Input: part model. Units: mm. Frame: model coordinates. Coordinates: 2 decimals unless noted, no trailing zeros. Write each loop counter-clockwise with the first axis right and the second up, starting at its lowest first coordinate (ties: lowest second). Pieces come first, ordered by that corner, then holes. Notation, with made-up numbers: (5, 29) - (54, 29) arc R17 cw to (54, 48) - close; hole circle Ø6 at (82, 3). An arc over 180 degrees is marked (long way). Put each result on its own line as item: value. Start each with the question number.
1. Cut plane B-B, the plane z = 6. Return loops of the section in (x, y).
2. Cut plane C-C, the plane x = 6. Return loops of the section in (y, z), and give its area (3 significant figures).
3. Cut plane A-A, the plane y = -13.5. Return loops of the section in (x, z).
4. Pin query (flat end, axial travel): pin 1 (1.5 mm diameter, centred on y = -30.5, z = 4.5, fed in from -X). Return the tip coordinate at first contact, or that it passes through.
5. Line query: line 1 (Z direction, x = -0.25, y = -7.5); line 2 (Z direction, x = 7.5, y = -33.5); line 3 (X direction, y = -27, z = 2.5). Output: solid intervals per line, ascending.
from build123d import *

# Parameters (mm, degrees)
F1_DEPTH = 40


with BuildPart() as f1:
    # F0 (on Front) → F1 (new body)
    with BuildSketch(Plane.XZ):
        with BuildLine():
            ThreePointArc((-6.6143782777, -7.5), (0, -10), (6.6143782777, -7.5))
            Line((6.6143782777, -7.5), (2.3e-08, -7.5))
            Line((2.3e-08, -7.5), (-6.6143782777, -7.5))
        make_face()
        with BuildLine():
            ThreePointArc((6.6143782777, -7.5), (9.1143782777, -4.1143782777), (10, 0))
            Line((10, 0), (7.5, 0))
            ThreePointArc((7.5, 0), (5.303300867, -5.3033008508), (2.3e-08, -7.5))
            Line((2.3e-08, -7.5), (6.6143782777, -7.5))
        make_face()
        with BuildLine():
            ThreePointArc((10, 0), (9.1143782777, 4.1143782777), (6.6143782777, 7.5))
            Line((6.6143782777, 7.5), (2.31e-08, 7.5))
            ThreePointArc((2.31e-08, 7.5), (5.3033008671, 5.3033008507), (7.5, 0))
            Line((7.5, 0), (10, 0))
        make_face()
        with BuildLine():
            Line((2.31e-08, 7.5), (6.6143782777, 7.5))
            ThreePointArc((6.6143782777, 7.5), (0, 10), (-6.6143782777, 7.5))
            Line((-6.6143782777, 7.5), (2.31e-08, 7.5))
        make_face()
        with BuildLine():
            ThreePointArc((-7.5, 0), (-5.3033008507, 5.3033008671), (2.31e-08, 7.5))
            Line((2.31e-08, 7.5), (-6.6143782777, 7.5))
            ThreePointArc((-6.6143782777, 7.5), (-9.1143782777, 4.1143782777), (-10, 0))
            Line((-10, 0), (-7.5, 0))
        make_face()
        with BuildLine():
            ThreePointArc((2.3e-08, -7.5), (-5.3033008508, -5.303300867), (-7.5, 0))
            Line((-7.5, 0), (-10, 0))
            ThreePointArc((-10, 0), (-9.1143782777, -4.1143782777), (-6.6143782777, -7.5))
            Line((-6.6143782777, -7.5), (2.3e-08, -7.5))
        make_face()
        with BuildLine():
            ThreePointArc((7.5, 0), (5.3033008671, 5.3033008507), (2.31e-08, 7.5))
            ThreePointArc((2.31e-08, 7.5), (-5.3033008507, 5.3033008671), (-7.5, 0))
            ThreePointArc((-7.5, 0), (-5.3033008508, -5.303300867), (2.3e-08, -7.5))
            ThreePointArc((2.3e-08, -7.5), (5.303300867, -5.3033008508), (7.5, 0))
        make_face()
    extrude(amount=F1_DEPTH)


solid = f1.part
Report:
1. outline: (-8, -40) - (8, -40) - (8, 0) - (-8, 0) - close
2. outline: (-40, -8) - (0, -8) - (0, 8) - (-40, 8) - close
2. area: 640 mm^2
3. outline: circle Ø20 at (0, 0)
4. pin 1: stops at x = -9.27
5. line 1: z = -10 to 10
5. line 2: z = -6.61 to 6.61
5. line 3: x = -9.68 to 9.68
